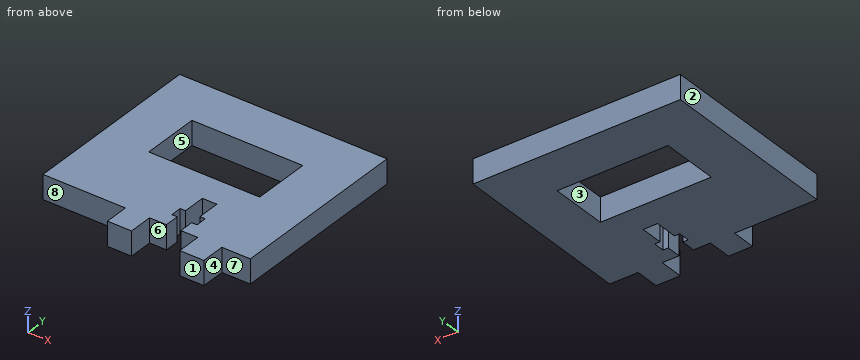
from build123d import *

# Parameters (mm, degrees)
SKETCH1_W           = 5
SKETCH1_H           = 5
SKETCH1_W_2         = 23
SKETCH1_H_2         = 12
BOSS_EXTRUDE3_DEPTH = 5


with BuildPart() as part:
    # Sketch1 → Boss-Extrude3 (new body)
    # profile 1 of 3: a face of its own
    with BuildSketch(Plane.XY):
        with Locations((-7.5, -24.5)):
            Rectangle(SKETCH1_W, SKETCH1_H)
    # profile 2 of 3: a face of its own
    with BuildSketch(Plane.XY):
        with Locations((7.5, -24.5)):
            Rectangle(SKETCH1_W, SKETCH1_H)
    # profile 3 of 3: a face of its own
    with BuildSketch(Plane.XY):
        Polygon((-27.1, 16), (-27.1, -22), (-10, -22), (-5, -22), (-1.5, -22), (-1.5, -19), (-2.6, -19), (-2.6, -16.7), (-1.5, -16.7), (-1.5, -12), (1.5, -12), (1.5, -16.7), (2.6, -16.7), (2.6, -19), (1.5, -19), (1.5, -22), (5, -22), (10, -22), (15.9, -22), (15.9, 16), align=None)
        with Locations((-5.6, 0)):
            Rectangle(SKETCH1_W_2, SKETCH1_H_2, mode=Mode.SUBTRACT)
    extrude(amount=BOSS_EXTRUDE3_DEPTH)


solid = part.part
Part model, mm, in its own coordinate system. Face numbers are marked on the shaded views. A direction names the side the tool comes from. Coordinates: 2 decimals unless noted, no trailing zeros. Loops run counter-clockwise (first coordinate to the right, second up) from the corner with the lowest first, then second, coordinate; pieces in that order, holes last. Notation, with made-up numbers: (63.25, 5.25) - (75.25, 5.25) arc R16 cw to (75.25, 26.25) - close; hole circle Ø5 at (65.25, 72). An arc over 180 degrees is marked (long way). Write each question's results on one line, items separated by ' | '. Start each with the question number.
Q1. Two-plate mould, pull along X, no slides. Class the marked faces 1, 2, 3 and 4: +X half, -X half, draft (parallel to the pull), parting line (faces both ways), or undercut.
Q2. Slice it at D-D on x = -22.5. Give the cut face in (y, z).
Q3. Probe line 1 along Y through (x, z) = (-5.5, 1); line 2 along Y through (x, z) = (0, 2.5); line 3 along X through (y, z) = (-17.5, 1.7). List the from-to ranges inside material, lowest first.
Q4. Drop flat-ended pins along their axis: pin 1 Ø1 at (x, z) = (-3.5, 3) entering from -Y; pin 2 Ø1.5 at (x, z) = (-0.5, 2) entering from -Y. Give the stop position or say it passes through.
Q5. Which spindle directions (+Z, -Z, +X, -X, +Y, -Y) get a long thin tool onto all of the face, cutting with end or side? Do the marked faces 5, 6, 7 and 8. Say none if no direction does.
Q6. Slice it at C-C on z = 2.25. Give the cut face in (x, y).
Q7. Slice it at B-B on x = 0.5. Give the cut face in (y, z), and give its area (3 significant figures).
Q8. Slice it at A-A on y = -2. Give the cut face in (x, z), and give its area (3 significant figures).
Answer:
1) face 1: draft | face 2: -X half | face 3: undercut | face 4: +X half
2) outline: (-22, 0) - (16, 0) - (16, 5) - (-22, 5) - close
3) line 1: y = -27 to -6, 6 to 16 | line 2: y = -12 to -6, 6 to 16 | line 3: x = -27.1 to -2.6, 2.6 to 15.9
4) pin 1: stops at y = -22 | pin 2: stops at y = -12
5) face 5: +Z, -Z | face 6: +Z, -Z, -Y | face 7: +Z, -Z, +X, -Y | face 8: +Z, -Z, -X, -Y
6) outline: (-27.1, -22) - (-10, -22) - (-10, -27) - (-5, -27) - (-5, -22) - (-1.5, -22) - (-1.5, -19) - (-2.6, -19) - (-2.6, -16.7) - (-1.5, -16.7) - (-1.5, -12) - (1.5, -12) - (1.5, -16.7) - (2.6, -16.7) - (2.6, -19) - (1.5, -19) - (1.5, -22) - (5, -22) - (5, -27) - (10, -27) - (10, -22) - (15.9, -22) - (15.9, 16) - (-27.1, 16) - close; hole (-17.1, -6) - (5.9, -6) - (5.9, 6) - (-17.1, 6) - close
7) outline: (-12, 0) - (-6, 0) - (-6, 5) - (-12, 5) - close; (6, 0) - (16, 0) - (16, 5) - (6, 5) - close | area: 80.0 mm2
8) outline: (-27.1, 0) - (-17.1, 0) - (-17.1, 5) - (-27.1, 5) - close; (5.9, 0) - (15.9, 0) - (15.9, 5) - (5.9, 5) - close | area: 100 mm2
